CAD build for the part. Positions are in the model's coordinates, mm. A direction names the side the tool comes from. Coordinates: 2 decimals unless noted, no trailing zeros. Loops run counter-clockwise (first coordinate to the right, second up) from the corner with the lowest first, then second, coordinate; pieces in that order, holes last. Notation, with made-up numbers: (33, -36) -> (48, -36) arc R10 cw to (48, -28) -> close; hole circle Ø9 at (-13.75, 35). An arc over 180 degrees is marked (long way). Answer as CSV lines item,"result". Start each with the question number.
```python
from build123d import *

# Parameters (mm, degrees)
SKETCH1_R           = 7
BOSS_EXTRUDE1_DEPTH = 9


with BuildPart() as part:
    # Sketch1 → Boss-Extrude1 (new body)
    with BuildSketch(Plane.XY):
        with BuildLine():
            Line((-139.941431307, -10.562383746), (-107.213509245, -7.990781577))
            ThreePointArc((-107.213509245, -7.990781577), (-105.245670948, -7.03654075), (-104.448510428, -5))
            Line((-104.448510428, -5), (-104.448510428, 5))
            ThreePointArc((-104.448510428, 5), (-105.245670948, 7.03654075), (-107.213509245, 7.990781577))
            Line((-107.213509245, 7.990781577), (-139.941431307, 10.562383746))
            ThreePointArc((-139.941431307, 10.562383746), (-142.212973239, 9.774441649), (-143.176432489, 7.571602169))
            Line((-143.176432489, 7.571602169), (-143.176432489, -7.571602169))
            ThreePointArc((-143.176432489, -7.571602169), (-142.212973239, -9.774441649), (-139.941431307, -10.562383746))
        make_face()
        with Locations((-133.176432489, 0)):
            Circle(SKETCH1_R, mode=Mode.SUBTRACT)
        with BuildLine():
            Line((-114.448510428, -6.5), (-120.448510428, -6.5))
            ThreePointArc((-120.448510428, -6.5), (-122.448510428, -4.5), (-120.448510428, -2.5))
            Line((-120.448510428, -2.5), (-114.448510428, -2.5))
            ThreePointArc((-114.448510428, -2.5), (-112.448510428, -4.5), (-114.448510428, -6.5))
        make_face(mode=Mode.SUBTRACT)
        with BuildLine():
            Line((-114.448510428, 2.5), (-120.448510428, 2.5))
            ThreePointArc((-120.448510428, 2.5), (-122.448510428, 4.5), (-120.448510428, 6.5))
            Line((-120.448510428, 6.5), (-114.448510428, 6.5))
            ThreePointArc((-114.448510428, 6.5), (-112.448510428, 4.5), (-114.448510428, 2.5))
        make_face(mode=Mode.SUBTRACT)
    extrude(amount=BOSS_EXTRUDE1_DEPTH)


solid = part.part
```
Q1. Which spindle directions (+Z, -Z, +X, -X, +Y, -Y) get a long thin tool onto all of the face, cutting with end or side? Do faces 4 (the flat face through (-123.807, -9.295, 4.437)), 5 (the flat face through (-117, -6.5, 4)). Say none if no direction does.
Q2. Saw through at C-C (x = -122). List the corners of the cut face in (y, z).
Q3. Saw through at A-A (y = 0). List the corners of the cut face in (x, z), and give its area (3 significant figures).
Q4. Probe probe 1 along X at (y, z) = (-4, 3.5) (3 decimals); probe 2 along Y at (x, z) = (-119, 3); probe 3 along X at (y, z) = (-5.25, 1). List the from-to ranges inside material, lowest first. Write a range as from..to.
Q5. Saw through at D-D (y = -3.25). List the corners of the cut face in (x, z), and give its area (3 significant figures).
Q6. Pin check, flat tips, straight feed: pin 1 Ø3 at (x, z) = (-116, 3.5) entering from -Y; pin 2 Ø3 at (x, z) = (-118.5, 3) entering from +Y; pin 3 Ø1.8 at (x, z) = (-117, 6.5) entering from +Y. Stop position of each tip, or through.
Q7. Two-plate mould, pull along X, no slides. Class faces 1 (the flat face through (-124, 0, 9)), 2 (the flat face through (-123.35, 9.26, 4.44)), 3 (the cylindrical face through (-126.5, 2.1, 4.4)): pulls with the +X half, pulls with the -X half, needs draft (parallel to the pull), parting line crosses it, or undercut.
Q8. Saw through at B-B (z = 3.75). List the corners of the cut face in (x, y).
Ans:
1,face 4,"+Z, -Z, +X, -Y"
1,face 5,"+Z, -Z"
2,outline,"(-9.15, 0) -> (-5.76, 0) -> (-5.76, 9) -> (-9.15, 9) -> close; (-3.24, 0) -> (3.24, 0) -> (3.24, 9) -> (-3.24, 9) -> close; (5.76, 0) -> (9.15, 0) -> (9.15, 9) -> (5.76, 9) -> close"
3,outline,"(-143.18, 0) -> (-140.18, 0) -> (-140.18, 9) -> (-143.18, 9) -> close; (-126.18, 0) -> (-104.45, 0) -> (-104.45, 9) -> (-126.18, 9) -> close"
3,area,"223 mm²"
4,probe 1,"x = -143.176..-138.921, -127.432..-122.385, -112.512..-104.449"
4,probe 2,"y = -8.92..-6.5, -2.5..2.5, 6.5..8.92"
4,probe 3,"x = -143.18..-137.81, -128.55..-122.3, -112.59..-104.46"
5,outline,"(-143.18, 0) -> (-139.38, 0) -> (-139.38, 9) -> (-143.18, 9) -> close; (-126.98, 0) -> (-122.01, 0) -> (-122.01, 9) -> (-126.98, 9) -> close; (-112.89, 0) -> (-104.45, 0) -> (-104.45, 9) -> (-112.89, 9) -> close"
5,area,"155 mm²"
6,pin 1,"stops at y = -8.8"
6,pin 2,"stops at y = 9"
6,pin 3,"stops at y = 8.83"
7,face 1,"needs draft"
7,face 2,"pulls with the +X half"
7,face 3,"undercut"
8,outline,"(-143.18, -7.57) arc R3 ccw to (-139.94, -10.56) -> (-107.21, -7.99) arc R3 ccw to (-104.45, -5) -> (-104.45, 5) arc R3 ccw to (-107.21, 7.99) -> (-139.94, 10.56) arc R3 ccw to (-143.18, 7.57) -> close; hole circle Ø14 at (-133.18, 0); hole (-120.45, -6.5) -> (-114.45, -6.5) arc R2 ccw to (-114.45, -2.5) -> (-120.45, -2.5) arc R2 ccw to start; hole (-120.45, 2.5) -> (-114.45, 2.5) arc R2 ccw to (-114.45, 6.5) -> (-120.45, 6.5) arc R2 ccw to start"
